from build123d import *

# Parameters (mm, degrees)
SKETCH1_R             = 17.5
BOSS_EXTRUDE1_DEPTH   = 5.5
SKETCH2_R             = 3.25
F_8_0MM_DOWEL_HOLE1_D = 8
F_4_0MM_DOWEL_HOLE1_D = 4


with BuildPart() as part:
    # Sketch1 → Boss-Extrude1 (new body, symmetric)
    with BuildSketch(Plane.XY):
        Circle(SKETCH1_R)
    extrude(amount=BOSS_EXTRUDE1_DEPTH, both=True)

    # Sketch2 → Cut-Revolve1 (revolve, cut)
    with BuildSketch(Plane(origin=(0, 0, 0), x_dir=(0, 0, -1), z_dir=(1, 0, 0))):
        with Locations((0, 18.5)):
            Circle(SKETCH2_R)
    revolve(axis=Axis((0, 0, 0), (0, 0, -1)), mode=Mode.SUBTRACT)

    # Ø8.0mm Dowel Hole1 (through all)
    with Locations(Plane.XY.offset(5.5)):
        with Locations((0, 0)):
            Hole(F_8_0MM_DOWEL_HOLE1_D / 2)

    # Ø4.0mm Dowel Hole1 (through all)
    with Locations(Plane.XY.offset(5.5)):
        with Locations((0, 12.7), (12.7, 0), (0, -12.7), (-12.7, 0)):
            Hole(F_4_0MM_DOWEL_HOLE1_D / 2)


solid = part.part
Here's how the part is built. I have some questions about the finished solid (model axes, mm). Coordinates: 2 decimals unless noted, no trailing zeros. Loops run counter-clockwise (first coordinate to the right, second up) from the corner with the lowest first, then second, coordinate; pieces in that order, holes last. Notation, with made-up numbers: (-26.5, -8) -> (15.5, -8) arc R24 ccw to (15.5, 29) -> close; hole circle Ø8 at (5.25, 41.5). An arc over 180 degrees is marked (long way). Use one line per item in the form item = value. Start each with the question number.
(1) Will these pins go through, and if not, where does the flat tip stop? pin 1 (4 mm diameter, centred on y = 3.5, z = 1.5, fed in from -X); pin 2 (6 mm diameter, centred on y = -7.5, z = -1.5, fed in from -X).
(2) We'd pull the mould along Y, two halves only. Please class faces 1 (the face through (-13.623, -1.774, -0.077)), 2 (the face through (-3.794, -17.084, -4.279)), 3 (the face through (4, -4, 5.5)): pulls with the +Y half, pulls with the -Y half, needs draft (parallel to the pull), parting line crosses it, or undercut.
(3) If we section it at C-C (z = 4.5): Please give me the cut outline in (x, y), then the cut area to 3 significant figures.
(4) If we section it at D-D (z = 1): Please give me the cut outline in (x, y).
(5) Please list where these lines run through material, in increasing order: line 1 along X through (y, z) = (0.5, 3.5); line 2 along X through (y, z) = (-1, 4.5); line 3 along X through (y, z) = (-11, 5.25).
(6) If we section it at A-A (x = 0): Please give me the cut outline in (y, z).
Verdict:
q1.pin_1 = -17.35
q1.pin_2 = -16.78
q2.face_1 = undercut
q2.face_2 = parting line crosses it
q2.face_3 = needs draft
q3.outline = circle Ø35 at (0, 0); hole circle Ø4 at (-12.7, 0); hole circle Ø8 at (0, 0); hole circle Ø4 at (0, -12.7); hole circle Ø4 at (0, 12.7); hole circle Ø4 at (12.7, 0)
q3.area = 862 mm²
q4.outline = circle Ø30.82 at (0, 0); hole circle Ø4 at (-12.7, 0); hole circle Ø8 at (0, 0); hole circle Ø4 at (0, -12.7); hole circle Ø4 at (0, 12.7); hole circle Ø4 at (12.7, 0)
q5.line_1 = -17.49 to -14.64, -10.76 to -3.97, 3.97 to 10.76, 14.64 to 17.49
q5.line_2 = -17.47 to -14.43, -10.97 to -3.87, 3.87 to 10.97, 14.43 to 17.47
q5.line_3 = -13.61 to -1.05, 1.05 to 13.61
q6.outline = (-17.5, -5.5) -> (-14.7, -5.5) -> (-14.7, 5.5) -> (-17.5, 5.5) -> (-17.5, 3.09) arc R3.25 cw to (-17.5, -3.09) -> close; (-10.7, -5.5) -> (-4, -5.5) -> (-4, 5.5) -> (-10.7, 5.5) -> close; (4, -5.5) -> (10.7, -5.5) -> (10.7, 5.5) -> (4, 5.5) -> close; (14.7, -5.5) -> (17.5, -5.5) -> (17.5, -3.09) arc R3.25 cw to (17.5, 3.09) -> (17.5, 5.5) -> (14.7, 5.5) -> close
